Autodesk Inventor part; units mm, degrees
ref_plane "Work Plane1" through (0, 0, -144) normal (0, 0, 1) x (1, 0, 0)
ref_plane "Work Plane2" through (340, 0, 0) normal (1, 0, 0) x (0, 0, -1)
ref_plane "YZ Plane" through (0, 0, 0) normal (1, 0, 0) x (0, 1, 0)
sketch "Sketch1" plane through (0, 0, 0) normal (0, 0, 1) x (1, 0, 0)
  line L0 (0, 0) -> (680, 0)
  line L1 (680, 0) -> (680, 350)
  line L2 (680, 350) -> (0, 350)
  line L3 (0, 350) -> (0, 0)
  line L4 (660, 20) -> (20, 20)
  line L5 (20, 20) -> (20, 330)
  line L6 (20, 330) -> (660, 330)
  line L7 (660, 330) -> (660, 20)
  dimension "d0" = 680
  dimension "d1" = 350
  dimension "d2" = 20
extrude "Extrusion1" add sketch "Sketch1" against normal blind 28
sketch "Sketch2" plane through (680, 0, 0) normal (1, 0, 0) x (0, 0, -1)
  line L0 (0, 350) -> (28, 350)
  line L1 (28, 350) -> (288, 350)
  line L2 (288, 350) -> (288, 0)
  line L3 (28, 350) -> (28, 0)
  line L4 (288, 0) -> (28, 0)
  line L5 (28, 330) -> (268, 330)
  line L6 (268, 330) -> (268, 20)
  line L7 (268, 20) -> (28, 20)
  point P0 (0, 0)
  dimension "d5" = 260
  dimension "d6" = 350
  dimension "d7" = 20
  dimension "d8" = 20
  dimension "d9" = 310
extrude "Extrusion2" add sketch "Sketch2" against normal blind 28 contours L1 L2 L4 L3 L7 L6 L5
ref_plane "Work Plane1" through (0, 0, -144) normal (0, 0, 1) x (1, 0, 0)
mirror "Mirror1" about plane through (0, 0, -144) normal (0, 0, 1) of "Extrusion1"
ref_plane "Work Plane2" through (340, 0, 0) normal (1, 0, 0) x (0, 0, -1)
mirror "Mirror2" about plane through (340, 0, 0) normal (1, 0, 0) of "Extrusion2"
sketch "Sketch4" plane through (0, 0, 0) normal (0, -1, 0) x (1, 0, 0)
  line L0 (0, -144) -> (680, -144)
  line L1 (680, -28) -> (680, -260)
  line L2 (680, -288) -> (0, -288)
  line L3 (0, -80.5) -> (680, -80.5)
  line L4 (652, -28) -> (28, -28)
  point P0 (0, 0)
  dimension "d15" = 144
  dimension "d16" = 52.5
properties part number "OuterShell" material "Steel, Mild"
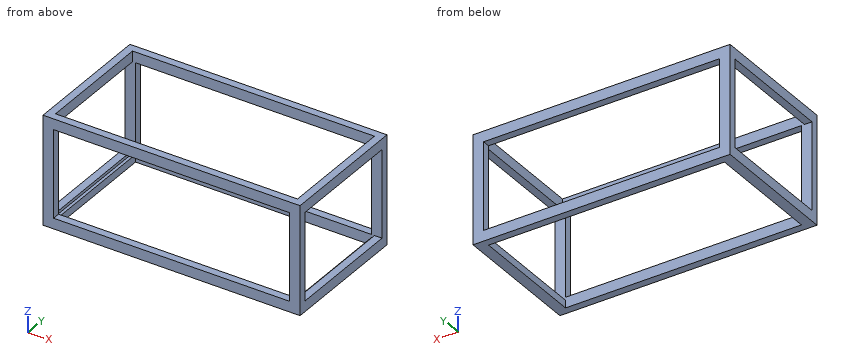
Read the model definition and answer for the solid it produces. Units are mm, in the model's axes. Give positions to 0.01 mm unless a question says otherwise; leave off trailing zeros. Write each loop counter-clockwise with the first axis right and the second up, starting at its lowest first coordinate (ties: lowest second). Pieces come first, ordered by that corner, then holes. Notation, with made-up numbers: (-15.75, -9.5) - (3.25, -9.5) arc R20 cw to (3.25, 6.5) - close; hole circle Ø4 at (57, 9.5). An arc over 180 degrees is marked (long way). Use CSV: the item, a comma, the result in double quotes. Start each with the question number.
(1) Consider line 1 along X through (y, z) = (19, -124); line 2 along Z through (x, y) = (111, 19.5); line 3 along Y through (x, z) = (535, -273.5). Determine where each line is inside the solid, lowest interval first.
(2) Find section B-B (y = 134). Give the vertices of the cut face in (x, z).
(3) Find section C-C (x = 637.5). Give the vertices of the cut face in (y, z).
(4) Given P1, Ø4, axis at x = 654, y = 241, coming from the +Z side, flat-ended and moving along its own axis, determine where the tip first touches the part or whether it passes through.
(5) Find section A-A (z = -67). Give the vertices of the cut face in (x, y).
Findings below:
1,line 1,"0 to 28, 652 to 680"
1,line 2,"-288 to -260, -28 to 0"
1,line 3,"0 to 20, 330 to 350"
2,outline,"(0, -288) - (28, -288) - (28, -268) - (20, -268) - (20, -260) - (0, -260) - close; (0, -28) - (20, -28) - (20, 0) - (0, 0) - close; (652, -288) - (680, -288) - (680, -260) - (660, -260) - (660, -268) - (652, -268) - close; (660, -28) - (680, -28) - (680, 0) - (660, 0) - close"
3,outline,"(0, -288) - (20, -288) - (20, -260) - (0, -260) - close; (0, -28) - (20, -28) - (20, 0) - (0, 0) - close; (330, -288) - (350, -288) - (350, -260) - (330, -260) - close; (330, -28) - (350, -28) - (350, 0) - (330, 0) - close"
4,P1,"z = -268"
5,outline,"(0, 0) - (28, 0) - (28, 20) - (0, 20) - close; (0, 330) - (28, 330) - (28, 350) - (0, 350) - close; (652, 0) - (680, 0) - (680, 20) - (652, 20) - close; (652, 330) - (680, 330) - (680, 350) - (652, 350) - close"
